```python
from build123d import *

# Parameters (mm, degrees)
SKETCH2_R           = 12.7
SKETCH6_R           = 15.24
BOSS_EXTRUDE2_DEPTH = 25.4
SKETCH7_R           = 15.24
CUT_EXTRUDE1_DEPTH  = 22.86


with BuildPart() as part:
    # Sweep1: sweep along a path in Sketch1
    with BuildLine(Plane(origin=(0, 0, 0), x_dir=(0, 0, -1), z_dir=(1, 0, 0))) as sweep1_path:
        Line((0, 0), (330.2, 0))
        Line((330.2, 0), (330.2, -152.4))
    # Sketch2 → Sweep1 (sweep)
    with BuildSketch(Plane.XY):
        Circle(SKETCH2_R)
    sweep(path=sweep1_path.line, transition=Transition.RIGHT)

    # Sketch6 → Boss-Extrude2 (add)
    with BuildSketch(Plane.XY):
        Circle(SKETCH6_R)
    extrude(amount=-BOSS_EXTRUDE2_DEPTH)

    # Sketch7 → Cut-Extrude1 (cut)
    with BuildSketch(Plane.XY):
        Circle(SKETCH7_R)
    extrude(amount=-CUT_EXTRUDE1_DEPTH, mode=Mode.SUBTRACT)


solid = part.part
```
Build history of the part. All positions in model axes, mm. A direction names the side the tool comes from. Round coordinates to 2 decimals unless told otherwise and drop trailing zeros. Write each loop counter-clockwise with the first axis right and the second up, starting at its lowest first coordinate (ties: lowest second). Pieces come first, ordered by that corner, then holes. Notation, with made-up numbers: (43.5, 22.25) -> (59.5, 22.25) arc R7 ccw to (59.5, 35.25) -> close; hole circle Ø7 at (26, -13.75). An arc over 180 degrees is marked (long way). Put each result on its own line as item: value.
Item 1: Slice it at A-A, the plane y = 0. Give the cut face in (x, z), plus the area to 3 significant figures.
Here are the results:
outline: (-15.24, -25.4) -> (-12.7, -25.4) -> (-12.7, -330.2) arc R12.7 ccw to (12.7, -330.2) -> (12.7, -25.4) -> (15.24, -25.4) -> (15.24, -22.86) -> (-15.24, -22.86) -> close
area: 8,070 mm^2
Item 2: Slice it at B-B, the plane x = 0. Give the cut face in (y, z).
Here are the results:
outline: (-152.4, -342.9) -> (12.7, -342.9) -> (12.7, -25.4) -> (15.24, -25.4) -> (15.24, -22.86) -> (-15.24, -22.86) -> (-15.24, -25.4) -> (-12.7, -25.4) -> (-12.7, -317.5) -> (-152.4, -317.5) -> close
Item 3: Two-plate mould, pull along Z, no slides. Class faces 1 (the face through (-3.3, -14.88, -24.11)), 2 (the face through (0, 0, -22.86)), 3 (the face through (-3.5, 12.5, -25.4)): pulls with the +Z half, pulls with the -Z half, needs draft (parallel to the pull), parting line crosses it, or undercut.
Here are the results:
face 1: needs draft
face 2: pulls with the +Z half
face 3: undercut
Item 4: Slice it at C-C, the plane z = -330.2. Give the cut face in (x, y), plus the area to 3 significant figures.
Here are the results:
outline: (-12.7, -152.4) -> (12.7, -152.4) -> (12.7, 0) arc R12.7 ccw to (-12.7, 0) -> close
area: 4,120 mm^2
Item 5: Slice it at D-D, the plane z = -296.5. Give the cut face in (x, y), plus the area to 3 significant figures.
Here are the results:
outline: circle Ø25.4 at (0, 0)
area: 507 mm^2
Item 6: Wall check: probe 1 along Y at (x, z) = (-1, -68.5); probe 2 along Y at (x, z) = (-6, -245.5); probe 3 along Z at (x, y) = (-9.5, -96). Give the ranges that are in metal, low to high. Write a range as from..to.
Here are the results:
probe 1: y = -12.66..12.66
probe 2: y = -11.19..11.19
probe 3: z = -338.63..-321.77
Item 7: Flat gauge pins, fed straight in: P1, Ø2, axis at x = -9, z = -199.5, coming from the +Y side; P2, Ø3, axis at x = -11.5, z = -77, coming from the +Y side; P3, Ø2, axis at x = -8, y = -24, coming from the -Z side. Where does each tip first touch, or does it go through?
Here are the results:
P1: stops at y = 9.86
P2: stops at y = 7.83
P3: stops at z = -340.8
Item 8: Tool access for faces 4 (the face through (-2.75, 12.4, -186.37)), 5 (the face through (5.86, -71.006, -341.467)), 6 (the face through (0, -152.4, -330)): list every direction of +Z, -Z, +X, -X, +Y, -Y with a clear straight run to the whole face (end or side of a thin tool).
Here are the results:
face 4: none
face 5: -Y
face 6: +Z, -Z, +X, -X, -Y
